Answer from the drawing. Dimensions are ordinates in mm from the lowest x, y and z of the part. A direction names the side the tool comes from. Round coordinates to 2 decimals unless told otherwise and drop trailing zeros. Write each loop counter-clockwise with the first axis right and the second up, starting at its lowest first coordinate (ties: lowest second). Pieces come first, ordered by that corner, then holes.
1. A tool of negligible diameter and unlimited length cuts with its end or side. For the marked faces 1 and 2, from which of +Z, -Z, +X, -X, +Y, -Y can it reach the whole face along a straight path? Write none if from no direction.
2. Find section C-C (x = 11). Write down the section's boundary in (y, z).
3. Straight lines are drawn through the part: probe 1 along X at (y, z) = (22, 1.15); probe 2 along Y at (x, z) = (12.25, 1.3); probe 3 along Y at (x, z) = (8, 1.9). For each, find the intervals that lie inside material, in ascending order.
4. Find section B-B (y = 10). Write down the section's boundary in (x, z).
5. Flat-ended cylindrical pins translate along their axes: pin 1 Ø0.7 at (y, z) = (16, 1.5) entering from -X; pin 2 Ø1 at (x, y) = (10.5, 17.5) entering from +Z; pin 3 Ø2 at (x, y) = (1.5, 5) entering from -Z; pin 4 Ø0.7 at (y, z) = (10.5, 1.5) entering from +X. Find the tip coordinate at first contact, or state that the pin passes through.
6. Find section A-A (z = 0.45). Write down the section's boundary in (x, y) (3 decimals), and give its area (4 significant figures).
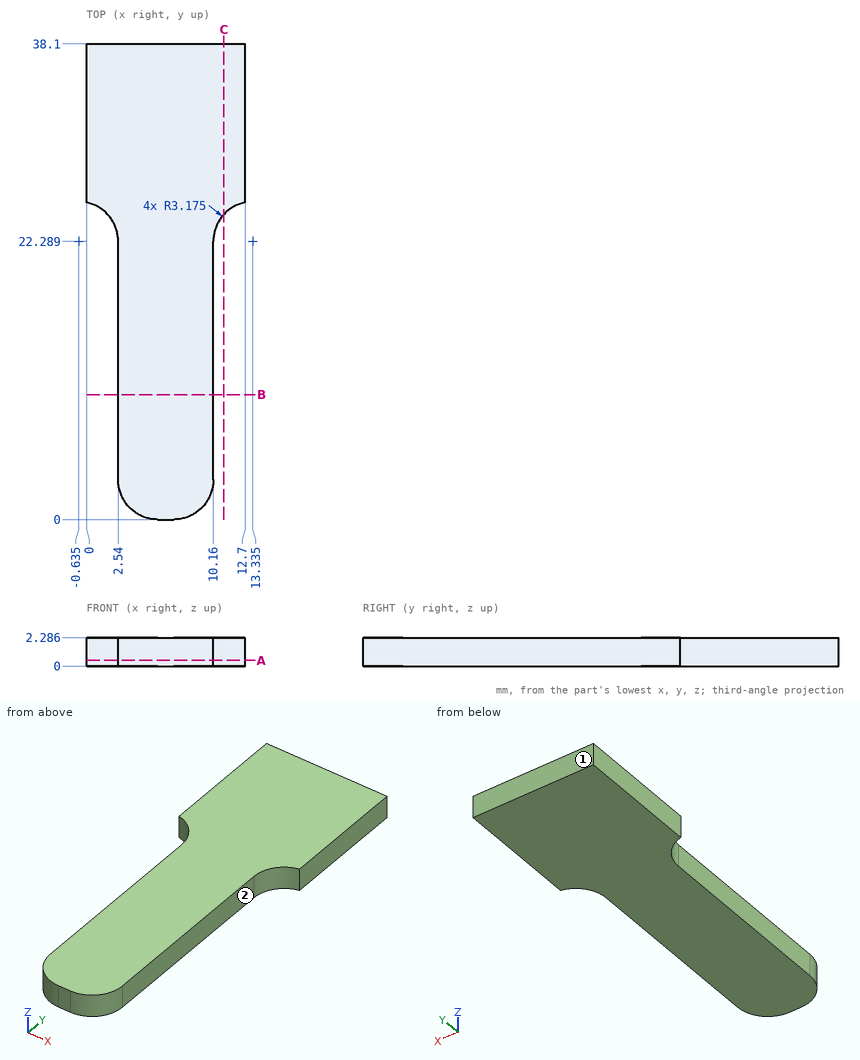
Worked answers:
1. face 1: +Z, -Z, +X, -X, +Y
1. face 2: +Z, -Z, +X, -Y
2. outline: (24.44, 0) - (38.1, 0) - (38.1, 2.29) - (24.44, 2.29) - close
3. probe 1: x = 2.54 to 10.16
3. probe 2: y = 25.27 to 38.1
3. probe 3: y = 0.17 to 38.1
4. outline: (2.54, 0) - (10.16, 0) - (10.16, 2.29) - (2.54, 2.29) - close
5. pin 1: stops at x = 2.54
5. pin 2: stops at z = 2.29
5. pin 3: passes through
5. pin 4: stops at x = 10.16
6. outline: (0, 25.4) arc R3.175 cw to (2.54, 22.289) - (2.54, 3.175) arc R3.175 ccw to (5.715, 0) - (6.985, 0) arc R3.175 ccw to (10.16, 3.175) - (10.16, 22.289) arc R3.175 cw to (12.7, 25.4) - (12.7, 38.1) - (0, 38.1) - close
6. area: 354.5 mm2
